```python
from build123d import *

# Parameters (mm, degrees)
SKETCH1_W                       = 159.7
SKETCH1_H                       = 109.7
SKETCH1_W_2                     = 130.9
SKETCH1_H_2                     = 88.7
BOSS_EXTRUDE1_DEPTH             = 20
SKETCH2_W                       = 143.7
SKETCH2_H                       = 102.7
SKETCH2_W_2                     = 130.9
SKETCH2_H_2                     = 88.7
CUT_EXTRUDE1_DEPTH              = 11.7
SKETCH3_W                       = 159.7
SKETCH3_H                       = 109.7
SKETCH3_W_2                     = 134.7
SKETCH3_H_2                     = 94.7
CUT_EXTRUDE2_DEPTH              = 5
FILLET1_R                       = 2
FILLET2_R                       = 8
M2X0_4_TAPPED_HOLE1_D           = 1.6
M2X0_4_TAPPED_HOLE1_DEPTH       = 3.5
M2X0_4_TAPPED_HOLE1_CSINK_D     = 2.05
M2X0_4_TAPPED_HOLE1_CSINK_ANGLE = 90
M2X0_4_TAPPED_HOLE1_TIP         = 0.480688495
SKETCH7_R                       = 2.7
BOSS_EXTRUDE2_DEPTH             = 5
SKETCH23_R                      = 1.75
BOSS_EXTRUDE5_DEPTH             = 5.5
SKETCH8_R                       = 1.9
BOSS_EXTRUDE3_DEPTH             = 2
SKETCH20_R                      = 1.25
BOSS_EXTRUDE4_DEPTH             = 10
CUT_EXTRUDE3_DEPTH              = 0.5
CUT_EXTRUDE4_DEPTH              = 12.5
SKETCH14_R                      = 1.1
CUT_EXTRUDE5_DEPTH              = 100.923946079
LPATTERN2_COUNT                 = 2
LPATTERN2_PITCH                 = 80
MIRROR6_COPY_1_DEPTH            = 12.5
MIRROR6_COPY_2_SKETCH_R         = 1.1
MIRROR6_COPY_2_DEPTH            = 100.923946079
FILLET4_R                       = 1
M3X0_5_TAPPED_HOLE1_D           = 2.5
M3X0_5_TAPPED_HOLE1_CSINK_D     = 3.05
M3X0_5_TAPPED_HOLE1_CSINK_ANGLE = 90
SKETCH18_R                      = 0.65
CUT_EXTRUDE6_DEPTH              = 0.5
SKETCH19_R                      = 1.4
CUT_EXTRUDE7_DEPTH              = 3.5
SKETCH24_R                      = 1
CUT_EXTRUDE8_DEPTH              = 0.5


with BuildPart() as part:
    # Sketch1 → Boss-Extrude1 (new body)
    with BuildSketch(Plane(origin=(0, 0, 0), x_dir=(1, 0, 0), z_dir=(0, 1, 0))):
        Rectangle(SKETCH1_W, SKETCH1_H)
        Rectangle(SKETCH1_W_2, SKETCH1_H_2, mode=Mode.SUBTRACT)
    extrude(amount=BOSS_EXTRUDE1_DEPTH)

    # Sketch2 → Cut-Extrude1 (cut)
    with BuildSketch(Plane(origin=(0, 20, 0), x_dir=(1, 0, 0), z_dir=(0, 1, 0))):
        Rectangle(SKETCH2_W, SKETCH2_H)
        Rectangle(SKETCH2_W_2, SKETCH2_H_2, mode=Mode.SUBTRACT)
    extrude(amount=-CUT_EXTRUDE1_DEPTH, mode=Mode.SUBTRACT)

    # Sketch3 → Cut-Extrude2 (cut)
    with BuildSketch(Plane.XZ):
        Rectangle(SKETCH3_W, SKETCH3_H)
        Rectangle(SKETCH3_W_2, SKETCH3_H_2, mode=Mode.SUBTRACT)
    extrude(amount=-CUT_EXTRUDE2_DEPTH, mode=Mode.SUBTRACT)

    # Fillet1
    fillet1_edges = [part.edges().sort_by_distance(p)[0] for p in [
        (-65.45, 4.15, 44.35),
        (65.45, 4.15, 44.35),
        (-65.45, 4.15, -44.35),
        (65.45, 4.15, -44.35),
        (71.85, 14.15, -51.35),
        (71.85, 14.15, 51.35),
        (-71.85, 14.15, 51.35),
        (-71.85, 14.15, -51.35),
    ]]
    fillet(fillet1_edges, radius=FILLET1_R)

    # Fillet2
    fillet2_edges = [part.edges().sort_by_distance(p)[0] for p in [
        (67.35, 2.5, -47.35),
        (-67.35, 2.5, -47.35),
        (-67.35, 2.5, 47.35),
        (67.35, 2.5, 47.35),
        (79.85, 12.5, 54.85),
        (-79.85, 12.5, 54.85),
        (-79.85, 12.5, -54.85),
        (79.85, 12.5, -54.85),
    ]]
    fillet(fillet2_edges, radius=FILLET2_R)

    # M2x0.4 Tapped Hole1
    with Locations(Plane(origin=(0, 20, 0), x_dir=(1, 0, 0), z_dir=(0, 1, 0))):
        with Locations((-77.5, 36), (-77.5, -36), (77.5, 36), (77.5, -36), (-74, 40), (-74, -40), (74, 40), (74, -40)):
            CounterSinkHole(M2X0_4_TAPPED_HOLE1_D / 2, M2X0_4_TAPPED_HOLE1_CSINK_D / 2, depth=M2X0_4_TAPPED_HOLE1_DEPTH, counter_sink_angle=M2X0_4_TAPPED_HOLE1_CSINK_ANGLE)
            with Locations((0, 0, -(M2X0_4_TAPPED_HOLE1_DEPTH + M2X0_4_TAPPED_HOLE1_TIP / 2))):  # 118° drill point
                Cone(0, M2X0_4_TAPPED_HOLE1_D / 2, M2X0_4_TAPPED_HOLE1_TIP, mode=Mode.SUBTRACT)

    # Sketch7 → Boss-Extrude2 (add)
    with BuildSketch(Plane(origin=(0, 20, 0), x_dir=(1, 0, 0), z_dir=(0, 1, 0))):
        with Locations(Location((-76.85, 44.85, 0), (0, 0, 270))):
            Circle(SKETCH7_R)
    extrude(amount=BOSS_EXTRUDE2_DEPTH)

    # Sketch23 → Boss-Extrude5 (add)
    with BuildSketch(Plane(origin=(0, 25, 0), x_dir=(1, 0, 0), z_dir=(0, 1, 0))):
        with Locations(Location((-76.85, 44.85, 0), (0, 0, 270))):
            Circle(SKETCH23_R)
    extrude(amount=BOSS_EXTRUDE5_DEPTH)

    # Sketch8 → Boss-Extrude3 (add)
    with BuildSketch(Plane(origin=(0, 20, 0), x_dir=(1, 0, 0), z_dir=(0, 1, 0))):
        with Locations(Location((-76.15, -51.15, 0), (0, 0, 270))):
            Circle(SKETCH8_R)
    extrude(amount=BOSS_EXTRUDE3_DEPTH)

    # Sketch20 → Boss-Extrude4 (add)
    with BuildSketch(Plane(origin=(0, 22, 0), x_dir=(1, 0, 0), z_dir=(0, 1, 0))):
        with Locations(Location((-76.15, -51.15, 0), (0, 0, 270))):
            Circle(SKETCH20_R)
    extrude(amount=BOSS_EXTRUDE4_DEPTH)

    # Sketch9 → Cut-Extrude3 (cut)
    with BuildSketch(Plane(origin=(0, 20, 0), x_dir=(1, 0, 0), z_dir=(0, 1, 0))):
        with BuildLine():
            Line((-74.85, 4), (-74.85, -4))
            ThreePointArc((-74.85, -4), (-76.85, -6), (-78.85, -4))
            Line((-78.85, -4), (-78.85, 4))
            ThreePointArc((-78.85, 4), (-76.85, 6), (-74.85, 4))
        make_face()
    cut_extrude3 = extrude(amount=-CUT_EXTRUDE3_DEPTH, mode=Mode.SUBTRACT)

    # Mirror1: Cut-Extrude3 across plane
    add(cut_extrude3.mirror(Plane(origin=(0, 0, 0), x_dir=(0, 0, 1), z_dir=(1, 0, 0))), mode=Mode.SUBTRACT)

    # Sketch11 → Cut-Extrude4 (cut)
    with BuildSketch(Plane(origin=(0, 20, 0), x_dir=(1, 0, 0), z_dir=(0, 1, 0))):
        with BuildLine():
            Line((-79.85, 42), (-79.85, 38))
            Line((-79.85, 38), (-77.5, 38))
            ThreePointArc((-77.5, 38), (-75.5, 40), (-77.5, 42))
            Line((-77.5, 42), (-79.85, 42))
        make_face()
    cut_extrude4 = extrude(amount=-CUT_EXTRUDE4_DEPTH, mode=Mode.SUBTRACT)

    # Sketch14 → Cut-Extrude5 (cut, through all)
    with BuildSketch(Plane(origin=(0, 7.5, 0), x_dir=(1, 0, 0), z_dir=(0, 1, 0))):
        with Locations(Location((-77.5, 40, 0), (0, 0, 270))):
            Circle(SKETCH14_R)
    cut_extrude5 = extrude(amount=-CUT_EXTRUDE5_DEPTH, mode=Mode.SUBTRACT)

    # LPattern2: Cut-Extrude4, Cut-Extrude5 ×2
    with Locations(*[(0, 0, i * LPATTERN2_PITCH) for i in range(1, LPATTERN2_COUNT)]):
        add(cut_extrude4, mode=Mode.SUBTRACT)
        add(cut_extrude5, mode=Mode.SUBTRACT)

    # Mirror6: Cut-Extrude4, Cut-Extrude5 across plane
    add(cut_extrude4.mirror(Plane(origin=(0, 0, 0), x_dir=(0, 0, 1), z_dir=(1, 0, 0))), mode=Mode.SUBTRACT)
    add(cut_extrude5.mirror(Plane(origin=(0, 0, 0), x_dir=(0, 0, 1), z_dir=(1, 0, 0))), mode=Mode.SUBTRACT)

    # Mirror6 copy 1 sketch → Mirror6 copy 1 (cut)
    with BuildSketch(Plane(origin=(0, 20, 80), x_dir=(-1, 0, 0), z_dir=(0, 1, 0))):
        with BuildLine():
            Line((-79.85, -42), (-79.85, -38))
            Line((-79.85, -38), (-77.5, -38))
            ThreePointArc((-77.5, -38), (-75.5, -40), (-77.5, -42))
            Line((-77.5, -42), (-79.85, -42))
        make_face()
    extrude(amount=-MIRROR6_COPY_1_DEPTH, mode=Mode.SUBTRACT)

    # Mirror6 copy 2 sketch → Mirror6 copy 2 (cut, through all)
    with BuildSketch(Plane(origin=(0, 7.5, 80), x_dir=(-1, 0, 0), z_dir=(0, 1, 0))):
        with Locations((-77.5, -40)):
            Circle(MIRROR6_COPY_2_SKETCH_R)
    extrude(amount=-MIRROR6_COPY_2_DEPTH, mode=Mode.SUBTRACT)

    # Fillet4
    fillet4_edges = [part.edges().sort_by_distance(p)[0] for p in [
        (-79.85, 13.75, -42),
        (-79.85, 13.75, -38),
        (-79.85, 13.75, 38),
        (-79.85, 13.75, 42),
        (79.85, 13.75, -42),
        (79.85, 13.75, -38),
        (79.85, 13.75, 38),
        (79.85, 13.75, 42),
    ]]
    fillet(fillet4_edges, radius=FILLET4_R)

    # M3x0.5 Tapped Hole1 (through all)
    with Locations(Plane(origin=(0, 20, 0), x_dir=(1, 0, 0), z_dir=(0, 1, 0))):
        with Locations((-77.5, 29), (-77.5, -29), (77.5, 29), (77.5, -29)):
            CounterSinkHole(M3X0_5_TAPPED_HOLE1_D / 2, M3X0_5_TAPPED_HOLE1_CSINK_D / 2, counter_sink_angle=M3X0_5_TAPPED_HOLE1_CSINK_ANGLE)

    # Sketch18 → Cut-Extrude6 (cut)
    with BuildSketch(Plane(origin=(0, 20, 0), x_dir=(1, 0, 0), z_dir=(0, 1, 0))):
        with Locations(Location((-77.85, 21.85, 0), (0, 0, 270))):
            Circle(SKETCH18_R)
    extrude(amount=-CUT_EXTRUDE6_DEPTH, mode=Mode.SUBTRACT)

    # Sketch19 → Cut-Extrude7 (cut)
    with BuildSketch(Plane(origin=(0, 20, 0), x_dir=(1, 0, 0), z_dir=(0, 1, 0))):
        with Locations(Location((77.35, 44.85, 0), (0, 0, 270))):
            Circle(SKETCH19_R)
        with Locations(Location((-77.35, -44.85, 0), (0, 0, 270))):
            Circle(SKETCH19_R)
    extrude(amount=-CUT_EXTRUDE7_DEPTH, mode=Mode.SUBTRACT)

    # Sketch24 → Cut-Extrude8 (cut)
    with BuildSketch(Plane(origin=(0, 8.3, 0), x_dir=(1, 0, 0), z_dir=(0, 1, 0))):
        with Locations(Location((68.45, -17.35, 0), (0, 0, 270))):
            Circle(SKETCH24_R)
    extrude(amount=-CUT_EXTRUDE8_DEPTH, mode=Mode.SUBTRACT)


solid = part.part
```
Input: part model. Units: mm. Frame: model coordinates. A direction names the side the tool comes from. Give positions to 0.01 mm unless a question says otherwise; leave off trailing zeros. Order: outer loops, then holes, each group sorted by start corner. A loop starts at its lowest first (then second) coordinate and runs counter-clockwise, first axis right, second up. Notation, with made-up numbers: M 4,39 L 27,39 A33 ccw 27,72 Z; hole C 7,10.25 d10. An arc over 180 degrees is marked long. Return JSON: item names as keys, results as strings.
1) Mould query, pull axis X, two halves, no side actions, for faces 1 (the face through (77, 19.5, 0)), 2 (the face through (-79, 7.5, -40)), 3 (the face through (65.069, 2.535, 44.944)). Classes: released by +X, released by -X, zero draft, split by the parting line, or undercut.
Taken from the geometry:
{"face 1": "undercut", "face 2": "zero draft", "face 3": "released by +X"}
2) Access query for faces 4 (the face through (-75.5, 13.8, -40)), 5 (the face through (-74.548, 20.986, 52.171)), 6 (the face through (79, 7.5, 40)). Directions: +Z, -Z, +X, -X, +Y, -Y. A direction counts if a zero-diameter tool reaches every point of the face in a straight line with its end or side. Return the directions, or none.
Taken from the geometry:
{"face 4": "-X, +Y", "face 5": "+Y", "face 6": "+X, +Y"}
3) Line query: L1, parallel to X at y = 15, z = 29; L2, parallel to X at y = 17.4, z = 36; L3, parallel to X at y = 8.15, z = 17.35. Output: solid intervals per line, ascending. Write a range as [from, to].
Taken from the geometry:
{"L1": "x = [-79.85, -78.75], [-76.25, -71.85], [71.85, 76.25], [78.75, 79.85]", "L2": "x = [-79.85, -78.3], [-76.7, -71.85], [71.85, 76.7], [78.3, 79.85]", "L3": "x = [-79.85, -65.45], [65.45, 67.45], [69.45, 79.85]"}
4) Contact query for flat-ended pins moving along their axis: pin 1 (2 mm diameter, centred on x = -78, z = -39.5, fed in from +Y); pin 2 (1.7 mm diameter, centred on x = 77.35, z = -44.85, fed in from +Y); pin 3 (1.4 mm diameter, centred on x = 74, z = 40, fed in from +Y); pin 4 (4 mm diameter, centred on x = -28.5, y = 3.5, fed in from +Z). Output: stop coordinate, or through.
Taken from the geometry:
{"pin 1": "stops at y = 7.5", "pin 2": "stops at y = 16.5", "pin 3": "stops at y = 16.44", "pin 4": "stops at z = 54.85"}
5) Section query B-B on y = 13. Count the separate pieces of the cut face and the enclosed holes in it, and give its area (3 significant figures).
Taken from the geometry:
{"separate pieces": "1", "enclosed holes": "5", "area": "2,630 mm2"}
6) Section query A-A on x = 46.5. Output: boundary loops of the cut face in (y, z), and give its area (3 significant figures).
Taken from the geometry:
{"outline": "M 0,-47.35 L 5,-47.35 L 5,-54.85 L 20,-54.85 L 20,-51.35 L 8.3,-51.35 L 8.3,-44.35 L 0,-44.35 Z; M 0,44.35 L 8.3,44.35 L 8.3,51.35 L 20,51.35 L 20,54.85 L 5,54.85 L 5,47.35 L 0,47.35 Z", "area": "181 mm2"}
